Can you work these out from the model? Positions are in its coordinate system, mm. Give positions to 0.01 mm unless a question says otherwise; leave off trailing zeros. Order: outer loops, then holes, each group sorted by start corner. A loop starts at its lowest first (then second) coordinate and runs counter-clockwise, first axis right, second up. Notation, with made-up numbers: M 37,4.5 L 62,4.5 A7 cw 62,16.5 Z; hole C 20,89 d7. An arc over 180 degrees is marked long. One line per question, with ' | ' between items. Start each with the question number.
1) Please list where these lines run through material, in increasing order: line 1 along X through (y, z) = (2.25, -46); line 2 along Z through (x, y) = (25.5, 2.25); line 3 along X through (y, z) = (4.75, -2). Write a range as [from, to].
2) If we section it at A-A, the plane z = -44.5: Please give me the cut outline in (x, y).
3) I'm going to push a flat-ended pin straight in: pin 1 Ø6 at (x, z) = (45, -45) entering from -Y. Where does the tip first touch, or does it pass through?
Autodesk Fusion 360 part; units mm, degrees
sketch "Sketch1" plane through (0, 0, 0) normal (0, 1, 0) x (1, 0, 0)
  line L0 (30, 50) -> (140, 50)
  line L1 (150, 40) -> (150, 10)
  line L2 (140, 0) -> (30, 0)
  line L3 (20, 10) -> (20, 40)
  arc A0 (150, 40) -> (140, 50) centre (140, 40) ccw
  arc A1 (140, 0) -> (150, 10) centre (140, 10) ccw
  arc A2 (30, 50) -> (20, 40) centre (30, 40) ccw
  arc A3 (20, 10) -> (30, 0) centre (30, 10) ccw
  point P0 (20, 50)
  point P1 (150, 50)
  point P2 (20, 0)
  dimension "d1" = 130
  dimension "d2" = 50
  dimension "d7" = 10
  dimension "d8" = 10
  dimension "d9" = 10
  dimension "d10" = 10
extrude "Extrude1" add sketch "Sketch1" along normal blind 6.35
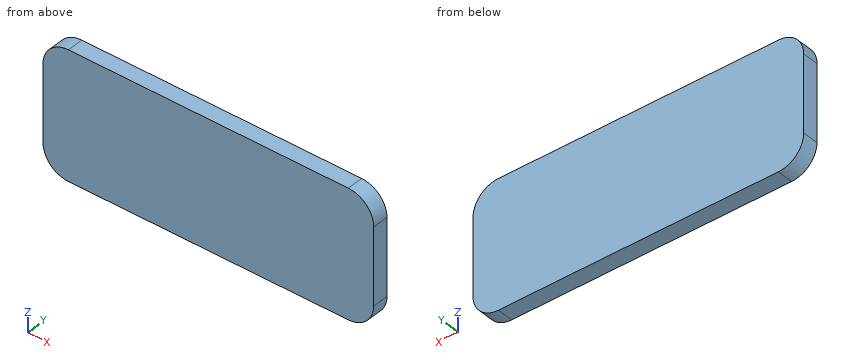
Results found:
1) line 1: x = [22, 148] | line 2: z = [-48.93, -1.07] | line 3: x = [24, 146]
2) outline: M 21.07,0 L 148.93,0 L 148.93,6.35 L 21.07,6.35 Z
3) pin 1: stops at y = 0
